Can you work these out from the model? Positions are in its coordinate system, mm. A direction names the side the tool comes from. Coordinates: 2 decimals unless noted, no trailing zeros. Loops run counter-clockwise (first coordinate to the right, second up) from the corner with the lowest first, then second, coordinate; pieces in that order, holes last. Notation, with made-up numbers: (13.25, -20.5) -> (64.25, -20.5) arc R12 ccw to (64.25, -12.5) -> close; hole circle Ø4 at (-19, 79.5). An arc over 180 degrees is marked (long way). Put each result on its own line as item: value. Start each with the question number.
Item 1: If we section it at C-C on z = 4.75: Please give me the cut outline in (x, y), plus the area to 3 significant figures.
Item 2: If we section it at D-D on x = -5.5: Please give me the cut outline in (y, z).
Item 3: Will these pins go through, and if not, where does the flat tip stop? P1, Ø2.5, axis at x = 12.37, y = 12.37, coming from the -Z side (1 decimal); P2, Ø3.5, axis at x = -20, z = 3.5, coming from the +Y side; P3, Ø2.5, axis at x = -20, z = 3.5, coming from the -Y side.
Item 4: We'd pull the mould along X, two halves only. Please class faces 1 (the cylindrical face through (13.3, 10.6, 3.5)), 2 (the flat face through (27.5, 0, 3)), 3 (the flat face through (0, 27.5, 3)): pulls with the +X half, pulls with the -X half, needs draft (parallel to the pull), parting line crosses it, or undercut.
Item 5: For faces 4 (the cylindrical face through (18.4, 23.1, 4.7)), 5 (the flat face through (-12, 0, 3)), 6 (the cylindrical face through (-21.998, -23.063, 3.588)), 7 (the flat face through (0, -27.5, 3)), which set-ups out of +Z, -Z, +X, -X, +Y, -Y let a thin tool reach every point of the face, with its end or its side?
Item 6: If we section it at A-A on y = -3: Please give me the cut outline in (x, z).
Item 7: Please list where these lines run through material, in increasing order: L1, parallel to Y at x = 12.5, z = 1.75; L2, parallel to X at y = -1, z = 3.25; L3, parallel to Z at x = 20, y = 21. Write a range as from..to.
Item 8: If we section it at B-B on x = 20: Please give me the cut outline in (y, z), plus the area to 3 significant figures.
```python
from build123d import *

# Parameters (mm, degrees)
SKETCH1_W           = 55
SKETCH1_H           = 55
SKETCH1_R           = 2
BOSS_EXTRUDE1_DEPTH = 7
SKETCH2_R           = 2
CUT_EXTRUDE1_DEPTH  = 9
SKETCH3_R           = 2
CUT_EXTRUDE2_DEPTH  = 9


with BuildPart() as part:
    # Sketch1 → Boss-Extrude1 (new body)
    with BuildSketch(Plane.XY):
        Rectangle(SKETCH1_W, SKETCH1_H)
        with Locations((-12.374368671, 12.374368671)):
            Circle(SKETCH1_R, mode=Mode.SUBTRACT)
        with Locations((12.374368671, 12.374368671)):
            Circle(SKETCH1_R, mode=Mode.SUBTRACT)
        with Locations((12.374368671, -12.374368671)):
            Circle(SKETCH1_R, mode=Mode.SUBTRACT)
        with Locations((-12.374368671, -12.374368671)):
            Circle(SKETCH1_R, mode=Mode.SUBTRACT)
        with BuildLine():
            Line((12, 5), (12, -5))
            ThreePointArc((12, -5), (0, -13), (-12, -5))
            Line((-12, -5), (-12, 5))
            ThreePointArc((-12, 5), (0, 13), (12, 5))
        make_face(mode=Mode.SUBTRACT)
    extrude(amount=BOSS_EXTRUDE1_DEPTH)

    # Sketch2 → Cut-Extrude1 (cut)
    with BuildSketch(Plane(origin=(0, 27.5, 0), x_dir=(1, 0, 0), z_dir=(0, 1, 0))):
        with Locations((-20, -3.5)):
            Circle(SKETCH2_R)
        with Locations((20, -3.5)):
            Circle(SKETCH2_R)
    extrude(amount=-CUT_EXTRUDE1_DEPTH, mode=Mode.SUBTRACT)

    # Sketch3 → Cut-Extrude2 (cut)
    with BuildSketch(Plane.XZ.offset(27.5)):
        with Locations((-20, 3.5)):
            Circle(SKETCH3_R)
        with Locations((20, 3.5)):
            Circle(SKETCH3_R)
    extrude(amount=-CUT_EXTRUDE2_DEPTH, mode=Mode.SUBTRACT)


solid = part.part
```
Solutions:
1. outline: (-27.5, -27.5) -> (-21.56, -27.5) -> (-21.56, -18.5) -> (-18.44, -18.5) -> (-18.44, -27.5) -> (18.44, -27.5) -> (18.44, -18.5) -> (21.56, -18.5) -> (21.56, -27.5) -> (27.5, -27.5) -> (27.5, 27.5) -> (21.56, 27.5) -> (21.56, 18.5) -> (18.44, 18.5) -> (18.44, 27.5) -> (-18.44, 27.5) -> (-18.44, 18.5) -> (-21.56, 18.5) -> (-21.56, 27.5) -> (-27.5, 27.5) -> close; hole circle Ø4 at (-12.37, -12.37); hole circle Ø4 at (-12.37, 12.37); hole (-12, -5) arc R13 ccw to (12, -5) -> (12, 5) arc R13 ccw to (-12, 5) -> close; hole circle Ø4 at (12.37, -12.37); hole circle Ø4 at (12.37, 12.37)
1. area: 2,340 mm^2
2. outline: (-27.5, 0) -> (-11.78, 0) -> (-11.78, 7) -> (-27.5, 7) -> close; (11.78, 0) -> (27.5, 0) -> (27.5, 7) -> (11.78, 7) -> close
3. P1: through
3. P2: y = 18.5
3. P3: y = -18.5
4. face 1: undercut
4. face 2: pulls with the +X half
4. face 3: needs draft
5. face 4: +Y
5. face 5: +Z, -Z
5. face 6: -Y
5. face 7: +Z, -Z, +X, -X, -Y
6. outline: (-27.5, 0) -> (-12, 0) -> (-12, 7) -> (-27.5, 7) -> close; (12, 0) -> (27.5, 0) -> (27.5, 7) -> (12, 7) -> close
7. L1: -27.5..-14.37, -10.38..10.38, 14.37..27.5
7. L2: -27.5..-12, 12..27.5
7. L3: 0..1.5, 5.5..7
8. outline: (-27.5, 0) -> (27.5, 0) -> (27.5, 1.5) -> (18.5, 1.5) -> (18.5, 5.5) -> (27.5, 5.5) -> (27.5, 7) -> (-27.5, 7) -> (-27.5, 5.5) -> (-18.5, 5.5) -> (-18.5, 1.5) -> (-27.5, 1.5) -> close
8. area: 313 mm^2
